Input: dimensioned drawing with shaded views. Units: mm. Origin: part minimum x, y, z. A direction names the side the tool comes from. Coordinates: 2 decimals unless noted, no trailing zeros. Order: outer loops, then holes, each group sorted by start corner. A loop starts at its lowest first (then second) coordinate and runs counter-clockwise, first axis right, second up. Notation, with made-up numbers: M -19,-37.75 L 13,-37.75 A25 ccw 13,-7.75 Z; hole C -30.5,35.5 d1. An arc over 180 degrees is marked long. Use CSV: the item, a comma, the result in double quotes. Start each with the question number.
1. Pull-direction query (X, two-part tool) for the marked faces 3, 4, 5 and 6; classes: pulls with the +X half, pulls with the -X half, needs draft (parallel to the pull), parting line crosses it, or undercut.
2. Section query A-A on x = 10. Return the cut outline in (y, z).
3. First-contact query: P1, Ø12, axis at y = 29, z = 23.5, coming from the +X side; P2, Ø12, axis at x = 6.5, z = 25, coming from the +Y side; P3, Ø5, axis at y = 16, z = 31.5, coming from the +X side. Flat tips, straight axial feed; report the tip coordinate or a pass-through.
4. Section query C-C on z = 33. Return the cut outline in (x, y) (1 decimal).
5. Section query B-B on y = 41. Return the cut outline in (x, z) (1 decimal), and give its area (3 significant figures).
6. Set-up query: the marked faces 1 and 2. Return all of +Z, -Z, +X, -X, +Y, -Y with unobstructed straight access to the full face (end or side cutting, diameter ignored); none if empty.
7. Material intervals for line 1 (Z direction, x = 22, y = 80.5); line 2 (Y direction, x = 34, z = 30) (1 decimal); line 3 (Z direction, x = 35, y = 20.5), sorted ascending.
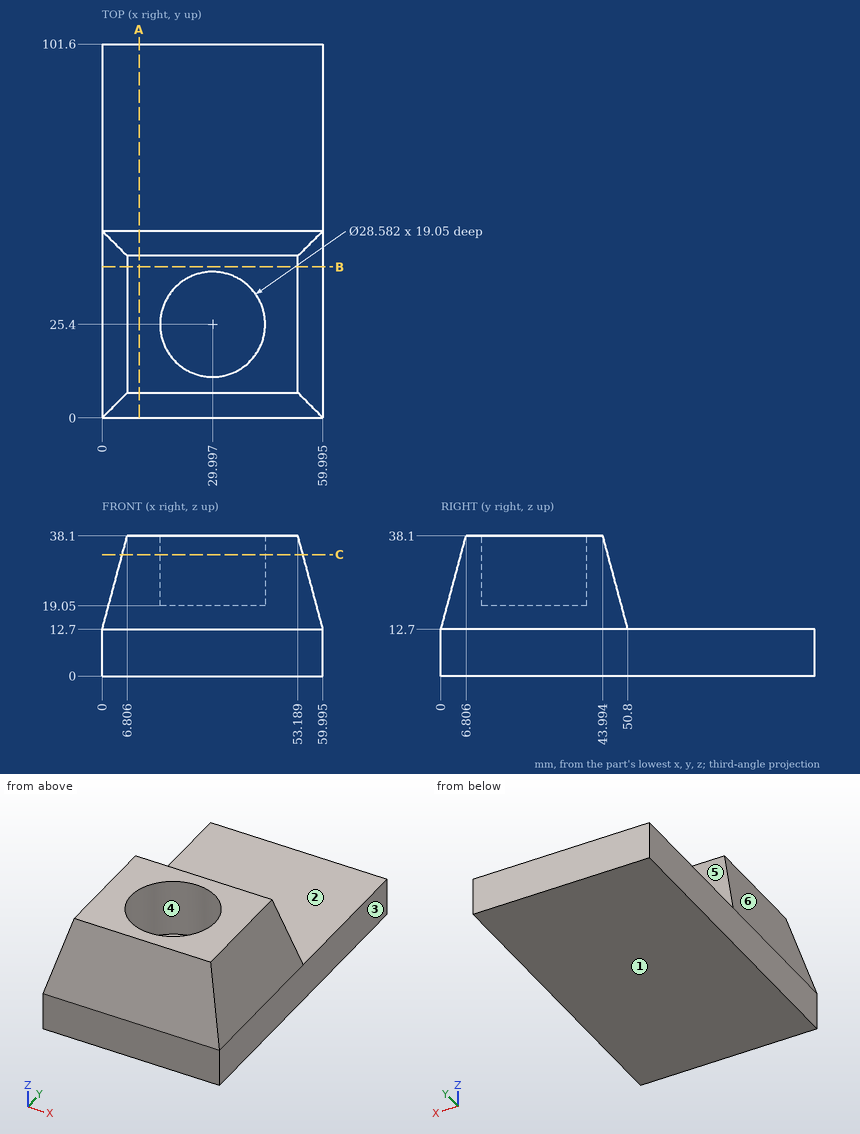
Results list:
1,face 3,"pulls with the +X half"
1,face 4,"undercut"
1,face 5,"needs draft"
1,face 6,"pulls with the -X half"
2,outline,"M 0,0 L 101.6,0 L 101.6,12.7 L 50.8,12.7 L 43.99,38.1 L 6.81,38.1 L 0,12.7 Z"
3,P1,"stops at x = 58.71"
3,P2,"stops at y = 49.11"
3,P3,"stops at x = 55.63"
4,outline,"M 5.4,5.4 L 54.6,5.4 L 54.6,45.4 L 5.4,45.4 Z; hole C 30,25.4 d28.6"
5,outline,"M 0,0 L 60,0 L 60,12.7 L 53.2,38.1 L 6.8,38.1 L 0,12.7 Z"
5,area,"2,110 mm²"
6,face 1,"-Z, +X, -X, +Y, -Y"
6,face 2,"+Z, +X, -X, +Y"
7,line 1,"z = 0 to 12.7"
7,line 2,"y = 4.6 to 11.7, 39.1 to 46.2"
7,line 3,"z = 0 to 19.05"
